Part print with two shaded views. Sizes in mm from the minimum x, y, z corner. A direction names the side the tool comes from. Coordinates: 2 decimals unless noted, no trailing zeros. Loops run counter-clockwise (first coordinate to the right, second up) from the corner with the lowest first, then second, coordinate; pieces in that order, holes last. Notation, with made-up numbers: (-20.75, 71.25) - (-14.75, 71.25) arc R24 ccw to (-14.75, 88.25) - close; hole circle Ø2 at (52, 72). An arc over 180 degrees is marked (long way). Answer as CSV lines item,"result".
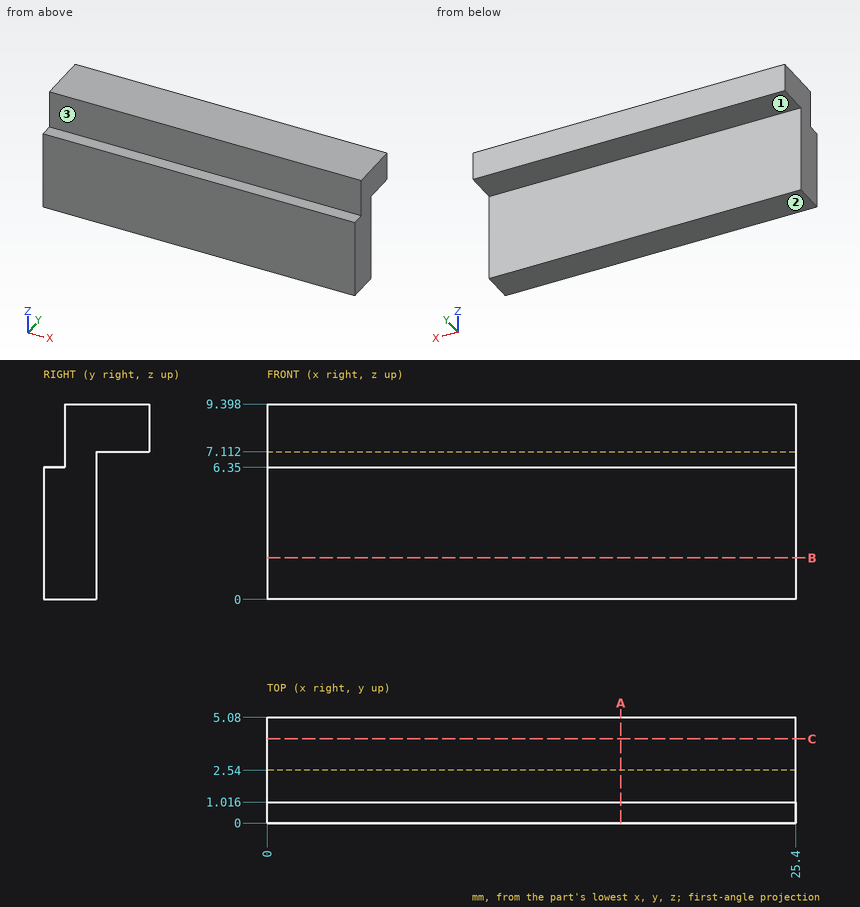
Q1. Saw through at C-C (y = 4.05). Give the cut face in (x, z), then the cut area to 3 significant figures.
Results:
outline,"(0, 7.11) - (25.4, 7.11) - (25.4, 9.4) - (0, 9.4) - close"
area,"58.1 mm^2"
Q2. Saw through at B-B (z = 2). Give the cut face in (x, y), then the cut area to 3 significant figures.
Results:
outline,"(0, 0) - (25.4, 0) - (25.4, 2.54) - (0, 2.54) - close"
area,"64.5 mm^2"
Q3. Flat gauge pins, fed straight in: pin 1 (1.1 mm diameter, centred on x = 18.5, y = 0.5, fed in from +Z); pin 2 (2 mm diameter, centred on x = 14.5, z = 2.5, fed in from +Y); pin 3 (1.5 mm diameter, centred on x = 18.5, z = 8, fed in from -Y). Where does each tip first touch, or does it go through?
Results:
pin 1,"stops at z = 9.4"
pin 2,"stops at y = 2.54"
pin 3,"stops at y = 1.02"
Q4. Wall check: L1, parallel to Z at x = 23, y = 2.6; L2, parallel to Y at x = 3.5, z = 2.25; L3, parallel to Y at x = 19.5, z = 7.5. Give the ranges that are in metal, low to high.
Results:
L1,"z = 7.11 to 9.4"
L2,"y = 0 to 2.54"
L3,"y = 1.02 to 5.08"
Q5. Which spindle directions (+Z, -Z, +X, -X, +Y, -Y) get a long thin tool onto all of the face, cutting with end or side? Do the marked faces 1, 2 and 3. Say none if no direction does.
Results:
face 1,"-Z, +X, -X, +Y"
face 2,"-Z, +X, -X, +Y, -Y"
face 3,"+Z, +X, -X, -Y"
Q6. Saw through at A-A (x = 17). Give the cut face in (y, z), then the cut area to 3 significant figures.
Results:
outline,"(0, 0) - (2.54, 0) - (2.54, 7.11) - (5.08, 7.11) - (5.08, 9.4) - (1.02, 9.4) - (1.02, 6.35) - (0, 6.35) - close"
area,"26.6 mm^2"
